from build123d import *

# Parameters (mm, degrees)
BOSS_EXTRUDE1_DEPTH = 6.35
SKETCH2_R           = 22.225
CUT_EXTRUDE1_DEPTH  = 6.35
FILLET2_R           = 3.175


with BuildPart() as part:
    # Sketch1 → Boss-Extrude1 (new body)
    with BuildSketch(Plane(origin=(0, 0, 0), x_dir=(1, 0, 0), z_dir=(0, 1, 0))):
        Polygon((359.098373018, -359.098373018), (490.5375, -131.439126982), (490.5375, 131.439126982), (359.098373018, 359.098373018), (131.439126982, 490.5375), (-131.439126982, 490.5375), (-359.098373018, 359.098373018), (-490.5375, 131.439126982), (-490.5375, -131.439126982), (-359.098373018, -359.098373018), (-131.439126982, -490.5375), (131.439126982, -490.5375), align=None)
    extrude(amount=BOSS_EXTRUDE1_DEPTH)

    # Sketch2 → Cut-Extrude1 (cut)
    with BuildSketch(Plane(origin=(0, 6.35, 0), x_dir=(1, 0, 0), z_dir=(0, 1, 0))):
        Circle(SKETCH2_R)
        Polygon((-131.439126982, 490.5375), (-197.430262751, 452.4375), (-47.625, 452.4375), (-47.625, 490.5375), align=None)
        Polygon((131.439126982, 490.5375), (47.625, 490.5375), (47.625, 452.4375), (197.430262751, 452.4375), align=None)
        with BuildLine():
            Line((3.3734375, 479.425), (3.3734375, 469.9))
            ThreePointArc((3.3734375, 469.9), (0, 466.5265625), (-3.3734375, 469.9))
            Line((-3.3734375, 469.9), (-3.3734375, 479.425))
            ThreePointArc((-3.3734375, 479.425), (0, 482.7984375), (3.3734375, 479.425))
        make_face()
        with BuildLine():
            Line((-50.8, 404.8125), (50.8, 404.8125))
            ThreePointArc((50.8, 404.8125), (66.675, 388.9375), (50.8, 373.0625))
            Line((50.8, 373.0625), (-50.8, 373.0625))
            ThreePointArc((-50.8, 373.0625), (-66.675, 388.9375), (-50.8, 404.8125))
        make_face()
        Polygon((401.005436509, 286.513209855), (359.098373018, 359.098373018), (293.107237249, 397.198373018), (368.009868625, 267.463209855), align=None)
        Polygon((490.5375, 55.239126982), (490.5375, 131.439126982), (448.630436509, 204.024290145), (415.634868625, 184.974290145), align=None)
        Polygon((448.630436509, -204.024290145), (490.5375, -131.439126982), (490.5375, -55.239126982), (415.634868625, -184.974290145), align=None)
        Polygon((293.107237249, -397.198373018), (359.098373018, -359.098373018), (401.005436509, -286.513209855), (368.009868625, -267.463209855), align=None)
        Polygon((47.625, -490.5375), (131.439126982, -490.5375), (197.430262751, -452.4375), (47.625, -452.4375), align=None)
        Polygon((-197.430262751, -452.4375), (-131.439126982, -490.5375), (-47.625, -490.5375), (-47.625, -452.4375), align=None)
        Polygon((-401.005436509, -286.513209855), (-359.098373018, -359.098373018), (-293.107237249, -397.198373018), (-368.009868625, -267.463209855), align=None)
        Polygon((-490.5375, -55.239126982), (-490.5375, -131.439126982), (-448.630436509, -204.024290145), (-415.634868625, -184.974290145), align=None)
        Polygon((-448.630436509, 204.024290145), (-490.5375, 131.439126982), (-490.5375, 55.239126982), (-415.634868625, 184.974290145), align=None)
        Polygon((-293.107237249, 397.198373018), (-359.098373018, 359.098373018), (-401.005436509, 286.513209855), (-368.009868625, 267.463209855), align=None)
        with BuildLine():
            Line((-413.507510459, 242.633982573), (-405.258618488, 237.871482573))
            ThreePointArc((-405.258618488, 237.871482573), (-404.023854665, 233.26328125), (-408.632055988, 232.028517427))
            Line((-408.632055988, 232.028517427), (-416.880947959, 236.791017427))
            ThreePointArc((-416.880947959, 236.791017427), (-418.115711782, 241.39921875), (-413.507510459, 242.633982573))
        make_face()
        with BuildLine():
            Line((416.880947959, 236.791017427), (408.632055988, 232.028517427))
            ThreePointArc((408.632055988, 232.028517427), (404.023854665, 233.26328125), (405.258618488, 237.871482573))
            Line((405.258618488, 237.871482573), (413.507510459, 242.633982573))
            ThreePointArc((413.507510459, 242.633982573), (418.115711782, 241.39921875), (416.880947959, 236.791017427))
        make_face()
        with BuildLine():
            Line((416.880947959, -236.791017427), (408.632055988, -232.028517427))
            ThreePointArc((408.632055988, -232.028517427), (404.023854665, -233.26328125), (405.258618488, -237.871482573))
            Line((405.258618488, -237.871482573), (413.507510459, -242.633982573))
            ThreePointArc((413.507510459, -242.633982573), (418.115711782, -241.39921875), (416.880947959, -236.791017427))
        make_face()
        with BuildLine():
            Line((-50.8, -404.8125), (50.8, -404.8125))
            ThreePointArc((50.8, -404.8125), (66.675, -388.9375), (50.8, -373.0625))
            Line((50.8, -373.0625), (-50.8, -373.0625))
            ThreePointArc((-50.8, -373.0625), (-66.675, -388.9375), (-50.8, -404.8125))
        make_face()
        with BuildLine():
            Line((3.3734375, -479.425), (3.3734375, -469.9))
            ThreePointArc((3.3734375, -469.9), (0, -466.5265625), (-3.3734375, -469.9))
            Line((-3.3734375, -469.9), (-3.3734375, -479.425))
            ThreePointArc((-3.3734375, -479.425), (0, -482.7984375), (3.3734375, -479.425))
        make_face()
        with BuildLine():
            Line((-413.507510459, -242.633982573), (-405.258618488, -237.871482573))
            ThreePointArc((-405.258618488, -237.871482573), (-404.023854665, -233.26328125), (-408.632055988, -232.028517427))
            Line((-408.632055988, -232.028517427), (-416.880947959, -236.791017427))
            ThreePointArc((-416.880947959, -236.791017427), (-418.115711782, -241.39921875), (-413.507510459, -242.633982573))
        make_face()
    extrude(amount=-CUT_EXTRUDE1_DEPTH, mode=Mode.SUBTRACT)

    # Fillet2
    fillet2_edges = [part.edges().sort_by_distance(p)[0] for p in [
        (-47.625, 3.175, 490.5375),
        (-197.430262751, 3.175, 452.4375),
        (-47.625, 3.175, 452.4375),
        (-293.107237249, 3.175, 397.198373018),
        (-401.005436509, 3.175, 286.513209855),
        (-368.009868625, 3.175, 267.463209855),
        (-448.630436509, 3.175, 204.024290145),
        (-490.5375, 3.175, 55.239126982),
        (-415.634868625, 3.175, 184.974290145),
        (-490.5375, 3.175, -55.239126982),
        (-448.630436509, 3.175, -204.024290145),
        (-415.634868625, 3.175, -184.974290145),
        (-401.005436509, 3.175, -286.513209855),
        (-293.107237249, 3.175, -397.198373018),
        (-368.009868625, 3.175, -267.463209855),
        (197.430262751, 3.175, 452.4375),
        (47.625, 3.175, 490.5375),
        (47.625, 3.175, 452.4375),
        (401.005436509, 3.175, 286.513209855),
        (293.107237249, 3.175, 397.198373018),
        (368.009868625, 3.175, 267.463209855),
        (490.5375, 3.175, 55.239126982),
        (448.630436509, 3.175, 204.024290145),
        (415.634868625, 3.175, 184.974290145),
        (448.630436509, 3.175, -204.024290145),
        (490.5375, 3.175, -55.239126982),
        (415.634868625, 3.175, -184.974290145),
        (293.107237249, 3.175, -397.198373018),
        (401.005436509, 3.175, -286.513209855),
        (368.009868625, 3.175, -267.463209855),
        (197.430262751, 3.175, -452.4375),
        (47.625, 3.175, -452.4375),
        (47.625, 3.175, -490.5375),
        (-47.625, 3.175, -490.5375),
        (-47.625, 3.175, -452.4375),
        (-197.430262751, 3.175, -452.4375),
    ]]
    fillet(fillet2_edges, radius=FILLET2_R)


solid = part.part
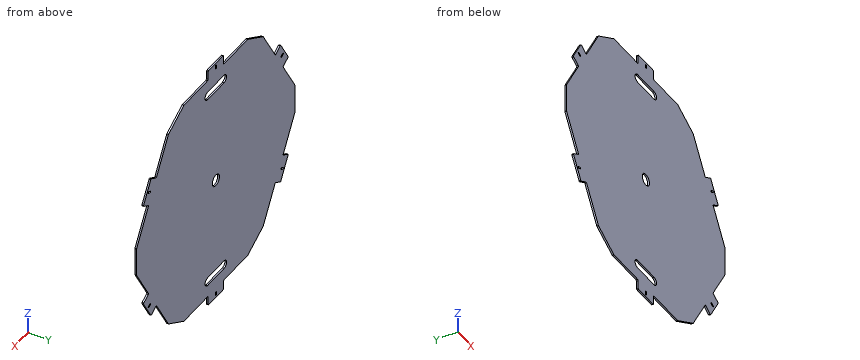
Design review of the part built by this model. Coordinates are the model's own, in mm. Give positions to 0.01 mm unless a question says otherwise; leave off trailing zeros. Loops run counter-clockwise (first coordinate to the right, second up) from the corner with the lowest first, then second, coordinate; pieces in that order, holes last. Notation, with made-up numbers: M -15.75,41.5 L 38.25,41.5 A25 ccw 38.25,72.5 Z; hole C -19.5,-13 d8. An arc over 180 degrees is marked long. Answer as a JSON object with one key per item and string values.
Item 1: Wall thickness on line 1 along Z through (x, y) = (-28.5, 1.25); line 2 along Z through (x, y) = (0, 3) (1 decimal); line 3 along X through (y, z) = (2.25, 0) (1 decimal): over which ranges is each line inside the solid? List them lowest first.
Output values:
{"line 1": "z = -490.54 to -404.81, -373.06 to 373.06, 404.81 to 490.54", "line 2": "z = -490.5 to -482.8, -466.5 to -404.8, -373.1 to -22.2, 22.2 to 373.1, 404.8 to 466.5, 482.8 to 490.5", "line 3": "x = -490.5 to -22.2, 22.2 to 490.5"}
Item 2: We need section B-B (y = 4). Count the separate pieces of the cut face and the enclosed holes in it, and give its area (3 significant figures).
Output values:
{"separate pieces": "1", "enclosed holes": "9", "area": "710,000 mm2"}
Item 3: For P1, Ø3, axis at x = 371, y = 2, coming from the +Z side; P2, Ø1.9, axis at x = -88.5, y = 3, coming from the -Z side; P3, Ø1.9, axis at y = 3, z = -473.5, coming from the +X side (3 decimals), all flat-tipped, find the tip position at first contact; note any pin that passes through.
Output values:
{"P1": "stops at z = 270.06", "P2": "stops at z = -452.44", "P3": "stops at x = 47.625"}
Item 4: We need section C-C (x = 131.5). State the section outline as (y, z) points, and give its area (3 significant figures).
Output values:
{"outline": "M 0,-452.44 L 6.35,-452.44 L 6.35,452.44 L 0,452.44 Z", "area": "5,750 mm2"}
Item 5: We need section D-D (z = 114). State the section outline as (x, y) points, and give its area (3 significant figures).
Output values:
{"outline": "M -456.61,0 L 456.61,0 L 456.61,6.35 L -456.61,6.35 Z", "area": "5,800 mm2"}
Item 6: We need section A-A (z = 384.5). State the section outline as (x, y) points, and give its area (3 significant figures).
Output values:
{"outline": "M -300.44,0 L -66.04,0 L -66.04,6.35 L -300.44,6.35 Z; M 66.04,0 L 300.44,0 L 300.44,6.35 L 66.04,6.35 Z", "area": "2,980 mm2"}
